from build123d import *

# Parameters (mm, degrees)
F0_W      = 50.8
F0_H      = 50.8
F1_DEPTH  = 38.1
F1_TAPER  = 30
F1_FACE_W = 50.8
F1_FACE_H = 50.8
F2_DEPTH  = 12.7
F2_TAPER  = 20
F3_R      = 18.4397946344
F4_DEPTH  = 101.6
F6_DEPTH  = 19.05
F7_DEPTH  = 19.05


with BuildPart() as f1:
    # F0 (on Top) → F1 (new body)
    with BuildSketch(Plane.XY):
        Rectangle(F0_W, F0_H)
    extrude(amount=-F1_DEPTH, taper=F1_TAPER)

    # F1_face (on face) → F2 (join)
    with BuildSketch(Plane.XY):
        Rectangle(F1_FACE_W, F1_FACE_H)
    extrude(amount=F2_DEPTH, taper=F2_TAPER)

    # F3 (on face) → F4 (join)
    with BuildSketch(Plane.XY.offset(12.7)):
        Circle(F3_R)
    extrude(amount=F4_DEPTH)

    # F5 (on Front) → F6 (join, symmetric)
    with BuildSketch(Plane.XZ):
        with BuildLine():
            Line((47.1632888286, 123.5673576593), (-47.1632888286, 123.5673576593))
            ThreePointArc((-47.1632888286, 123.5673576593), (-65.0582543601, 130.9796950807), (-57.6459169388, 113.0847295492))
            Line((-57.6459169388, 113.0847295492), (-57.6459169388, 106.2794923782))
            Line((-57.6459169388, 106.2794923782), (57.6459169388, 106.2794923782))
            Line((57.6459169388, 106.2794923782), (57.6459169388, 113.0847295492))
            ThreePointArc((57.6459169388, 113.0847295492), (65.0582543601, 130.9796950807), (47.1632888286, 123.5673576593))
        make_face()
    extrude(amount=F6_DEPTH, both=True)

    # F5 (on Front) → F7 (join, symmetric)
    with BuildSketch(Plane.XZ):
        with BuildLine():
            Line((47.1632888286, 123.5673576593), (-47.1632888286, 123.5673576593))
            ThreePointArc((-47.1632888286, 123.5673576593), (-65.0582543601, 130.9796950807), (-57.6459169388, 113.0847295492))
            Line((-57.6459169388, 113.0847295492), (-57.6459169388, 106.2794923782))
            Line((-57.6459169388, 106.2794923782), (57.6459169388, 106.2794923782))
            Line((57.6459169388, 106.2794923782), (57.6459169388, 113.0847295492))
            ThreePointArc((57.6459169388, 113.0847295492), (65.0582543601, 130.9796950807), (47.1632888286, 123.5673576593))
        make_face()
    extrude(amount=F7_DEPTH, both=True)


solid = f1.part
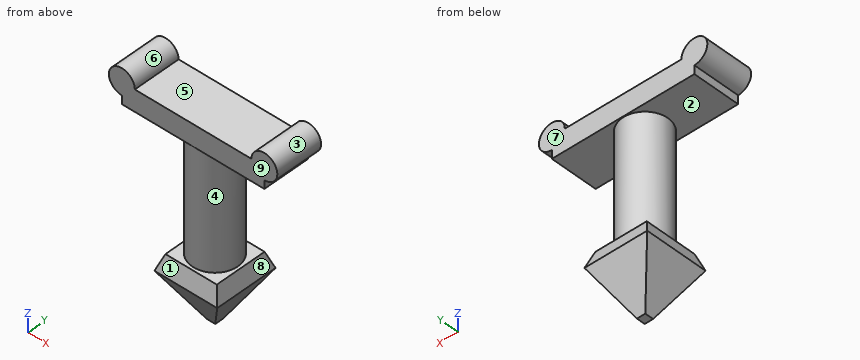
Read the model definition and answer for the solid it produces. Units are mm, in the model's axes. Face numbers are marked on the shaded views. A direction names the side the tool comes from. Coordinates: 2 decimals unless noted, no trailing zeros. Order: outer loops, then holes, each group sorted by start corner. A loop starts at its lowest first (then second) coordinate and runs counter-clockwise, first axis right, second up. Notation, with made-up numbers: M 42,26 L 75,26 A24 cw 75,56 Z; hole C -28.75,89.5 d7. An arc over 180 degrees is marked long. Put each result on its own line as item: value. Start each with the question number.
Item 1: Consider probe 1 along Z at (x, y) = (-25.5, 9.5); probe 2 along Y at (x, z) = (59, 123.5); probe 3 along Z at (x, y) = (19, 10.5). Determine where each line is inside the solid, lowest interval first. Write a range as [from, to].
Item 2: For the marked faces 5, 6, 7, 8 and 9, determine the directions among +Z, -Z, +X, -X, +Y, -Y from which every point of the face is accessible in a straight line to the end or side of a thin tool.
Item 3: Given pin 1 Ø12.5 at (x, y) = (-7, 3.5) entering from +Z; pin 2 Ø3.5 at (y, z) = (-0.5, 108.5) entering from +X; pin 3 Ø8.5 at (x, z) = (-2, 118.5) entering from +Y; pin 4 Ø12 at (x, z) = (32, 12) entering from +Y, each flat-ended and moving along its own axis, determine where each tip first touches the part or whether it passes through.
Item 4: Section A-A, the plane x = 33 is taken. Determine the outline of the cut face in (y, z), plus the area to 3 significant figures.
Item 5: Section B-B, the plane z = 98 is taken. Determine the outline of the cut face in (x, y), plus the area to 3 significant figures.
Item 6: The mould has two halves that part along Z. Classify the marked faces 1, 2, 3 and 4: +Z half, -Z half, draft (parallel to the pull), parting line (faces both ways), or undercut.
Computed:
1. probe 1: z = [106.28, 123.57]
1. probe 2: y = [-19.05, 19.05]
1. probe 3: z = [-11.09, 12.7], [106.28, 123.57]
2. face 5: +Z, +Y, -Y
2. face 6: +Y, -Y
2. face 7: +Z, +X, -X, +Y
2. face 8: +X, +Y, -Y
2. face 9: +Z, +X, -X, -Y
3. pin 1: stops at z = 123.57
3. pin 2: stops at x = 57.65
3. pin 3: stops at y = 19.05
3. pin 4: passes through
4. outline: M -19.05,106.28 L 19.05,106.28 L 19.05,123.57 L -19.05,123.57 Z
4. area: 659 mm2
5. outline: C 0,0 d36.88
5. area: 1,070 mm2
6. face 1: +Z half
6. face 2: undercut
6. face 3: parting line
6. face 4: undercut
